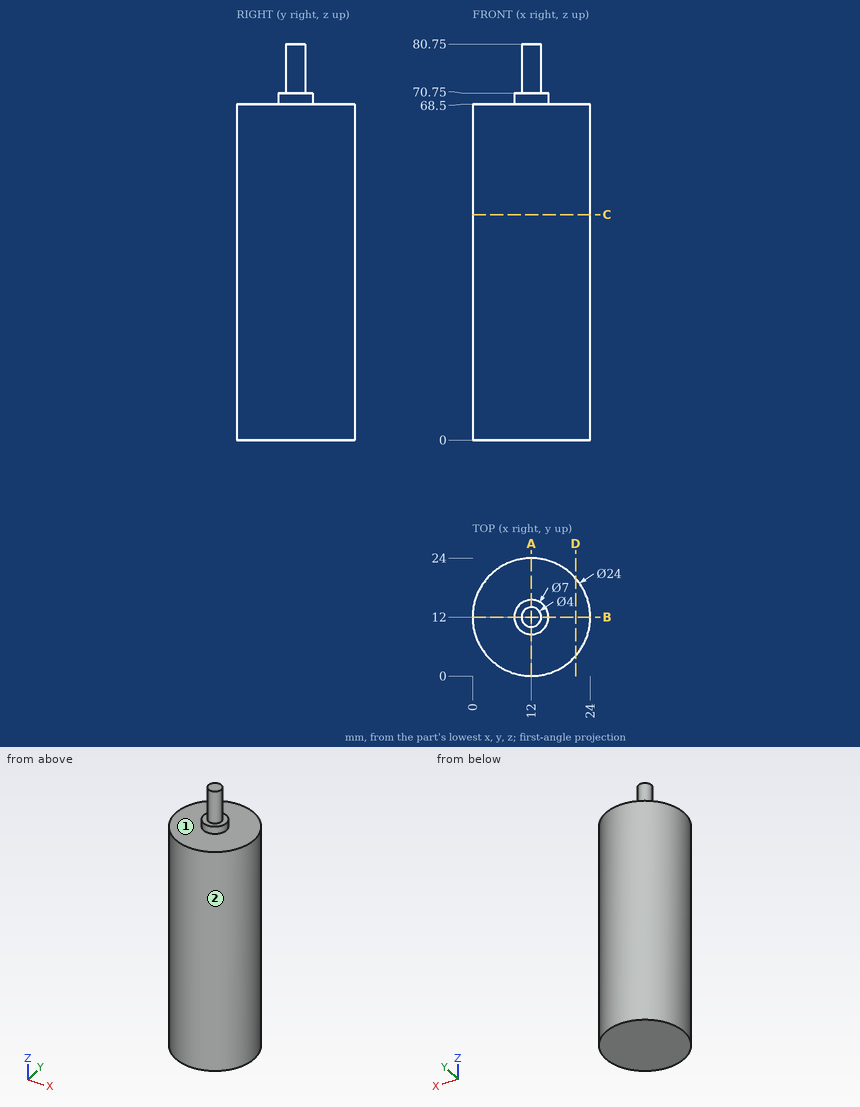
The drawing under review shows one solid part. Ordinate dimensions are in mm from its lowest x, y, z. A direction names the side the tool comes from. Round coordinates to 2 decimals unless told otherwise and drop trailing zeros. Write each loop counter-clockwise with the first axis right and the second up, starting at its lowest first coordinate (ties: lowest second). Pieces come first, ordered by that corner, then holes.
(1) We need section D-D on x = 21. Give the boundary of the cut face in (y, z), and give its area (3 significant figures).
(2) Insertion check: pin 1 (6 mm diameter, centred on x = 6.5, z = 58.5, fed in from -Y); pin 2 (2 mm diameter, centred on y = 7, z = 11.5, fed in from +X); pin 3 (1.5 mm diameter, centred on y = 4.5, z = 20.5, fed in from +X); pin 4 (1.5 mm diameter, centred on x = 2.5, y = 5.5, fed in from -Z). Each pin has a flat end and moves straight along its axis. Give the tip position at first contact, or say it passes through.
(3) We need section C-C on z = 46. Give the boundary of the cut face in (x, y), and give its area (3 significant figures).
(4) Wall thickness on L1, parallel to Z at x = 21.25, y = 5.25; L2, parallel to X at y = 12.5, z = 54.5; L3, parallel to Y at x = 11.75, z = 50.5: over which ranges is each line inside the solid? List them lowest first.
(5) We need section A-A on x = 12. Give the boundary of the cut face in (y, z), and give its area (3 significant figures).
(6) Machinability: for the marked faces 1 and 2, which of the approach directions +Z, -Z, +X, -X, +Y, -Y give a long, thin tool a straight path to every point of the face, cutting with its end or side? Answer none if there is none.
Findings below:
1. outline: (4.06, 0) - (19.94, 0) - (19.94, 68.5) - (4.06, 68.5) - close
1. area: 1,090 mm2
2. pin 1: stops at y = 0.26
2. pin 2: stops at x = 23.31
2. pin 3: stops at x = 21.92
2. pin 4: stops at z = 0
3. outline: circle Ø24 at (12, 12)
3. area: 452 mm2
4. L1: z = 0 to 68.5
4. L2: x = 0.01 to 23.99
4. L3: y = 0 to 24
5. outline: (0, 0) - (24, 0) - (24, 68.5) - (15.5, 68.5) - (15.5, 70.75) - (14, 70.75) - (14, 80.75) - (10, 80.75) - (10, 70.75) - (8.5, 70.75) - (8.5, 68.5) - (0, 68.5) - close
5. area: 1,700 mm2
6. face 1: +Z
6. face 2: +Z, -Z
